```python
from build123d import *

# Parameters (mm, degrees)
F0_R      = 10
F1_DEPTH  = 2.5
F2_R      = 7.5
F3_DEPTH  = 10
F4_R      = 7.15
F5_DEPTH  = 1.5
F6_R      = 7.5
F7_DEPTH  = 16.5
F8_R      = 6
F9_DEPTH  = 20
F10_SIZE  = 1
F11_R     = 7.75
F12_DEPTH = 15
F13_R     = 2.75
F14_DEPTH = 42
F15_SIZE  = 1
F16_R     = 1.5
F17_DEPTH = 12.5
F19_DEPTH = 6
F20_DEPTH = 4.2


with BuildPart() as f1:
    # F0 (on Front) → F1 (new body, symmetric)
    with BuildSketch(Plane.XZ):
        Circle(F0_R)
    extrude(amount=F1_DEPTH, both=True)

    # F2 (on face) → F3 (join)
    with BuildSketch(Plane.XZ.offset(2.5)):
        Circle(F2_R)
    extrude(amount=F3_DEPTH)

    # F4 (on face) → F5 (join)
    with BuildSketch(Plane.XZ.offset(12.5)):
        Circle(F4_R)
    extrude(amount=F5_DEPTH)

    # F6 (on face) → F7 (join)
    with BuildSketch(Plane.XZ.offset(14)):
        Circle(F6_R)
    extrude(amount=F7_DEPTH)

    # F8 (on face) → F9 (join)
    with BuildSketch(Plane.XZ.offset(30.5)):
        Circle(F8_R)
    extrude(amount=F9_DEPTH)

    # F10
    f10_edges = [f1.edges().sort_by_distance(p)[0] for p in [
        (-6, -50.5, 0),
    ]]
    chamfer(f10_edges, length=F10_SIZE)

    # F11 (on face) → F12 (join)
    with BuildSketch(Plane(origin=(0, 2.5, 0), x_dir=(-1, 0, 0), z_dir=(0, 1, 0))):
        Circle(F11_R)
    extrude(amount=F12_DEPTH)

    # F13 (on face) → F14 (join)
    with BuildSketch(Plane(origin=(0, 17.5, 0), x_dir=(-1, 0, 0), z_dir=(0, 1, 0))):
        Circle(F13_R)
    extrude(amount=F14_DEPTH)

    # F15
    f15_edges = [f1.edges().sort_by_distance(p)[0] for p in [
        (2.75, 59.5, 0),
    ]]
    chamfer(f15_edges, length=F15_SIZE)

    # F16 (on Top) → F17 (cut, symmetric)
    with BuildSketch(Plane.XY):
        with Locations((0, 14.5)):
            Circle(F16_R)
    extrude(amount=F17_DEPTH, both=True, mode=Mode.SUBTRACT)

    # F18 (on Top) → F19 (cut)
    with BuildSketch(Plane.XY):
        with BuildLine():
            Line((-1.5, -34), (-1.5, -50.5))
            Line((-1.5, -50.5), (1.5, -50.5))
            Line((1.5, -50.5), (1.5, -34))
            ThreePointArc((1.5, -34), (1.06066, -32.93934), (0, -32.5))
            ThreePointArc((0, -32.5), (-1.06066, -32.93934), (-1.5, -34))
        make_face()
    extrude(amount=F19_DEPTH, mode=Mode.SUBTRACT)

    # F18 (on Top) → F20 (join)
    with BuildSketch(Plane.XY):
        with BuildLine():
            Line((-1.5, -34), (-1.5, -50.5))
            Line((-1.5, -50.5), (1.5, -50.5))
            Line((1.5, -50.5), (1.5, -34))
            ThreePointArc((1.5, -34), (1.06066, -32.93934), (0, -32.5))
            ThreePointArc((0, -32.5), (-1.06066, -32.93934), (-1.5, -34))
        make_face()
    extrude(amount=F20_DEPTH)


solid = f1.part
```
CAD build for the part. Positions are in the model's coordinates, mm. A direction names the side the tool comes from. Round coordinates to 2 decimals unless told otherwise and drop trailing zeros. Loops run counter-clockwise (first coordinate to the right, second up) from the corner with the lowest first, then second, coordinate; pieces in that order, holes last. Notation, with made-up numbers: M 34.5,22.5 L 71.5,22.5 A27 cw 71.5,46.5 Z; hole C 81.5,15 d4. An arc over 180 degrees is marked long. Return JSON: item names as keys, results as strings. Group by question number.
(1) Drop flat-ended pins along their axis: P1, Ø0.8, axis at y = -39, z = 5, coming from the +X side; P2, Ø12, axis at x = -6.5, y = 18, coming from the -Z side; P3, Ø2.5, axis at x = 0.5, y = -44, coming from the +Z side; P4, Ø1, axis at x = 4, y = 28.5, coming from the -Z side. Give the stop position or say it passes through.
(2) Wall check: probe 1 along X at (y, z) = (14.5, -2); probe 2 along Y at (x, z) = (0, -3); probe 3 along Y at (x, z) = (0, -1). Give the ranges that are in metal, low to high. Write a range as [from, to].
(3) Mould opens along Y. For faces 5 (the flat face through (2, -30.5, 6)), 6 (the cylindrical face through (-0.93, -13.24, 7.09)), 7 (the cylindrical face through (-2.17, -0.04, -9.76)) say: +Y half, -Y half, draft (parallel to the pull), parting line (faces both ways), or undercut.
(4) Tool access for faces 1 (the flat face through (0, -41, 4.2)), 2 (the cylindrical face through (1.68, 9.895, -7.566)), 3 (the flat face through (0, 59.5, 0)), 4 (the flat face through (4, -2.5, 7)): list every direction of +Z, -Z, +X, -X, +Y, -Y with a clear straight run to the whole face (end or side of a thin tool).
(5) Saw through at A-A, the plane y = 14.5. List the corners of the cut face in (x, z), and give its area (3 significant figures).
(6) Saw through at B-B, the plane y = -7. List the corners of the cut face in (x, z).
Answer list:
{
 "1": {"P1": "x = 3.85", "P2": "z = -7.73", "P3": "z = 5.81", "P4": "through"},
 "2": {"probe 1": "[-7.49, -1.5], [1.5, 7.49]", "probe 2": "[-50.5, 13], [16, 17.5]", "probe 3": "[-50.5, 13], [16, 59.5]"},
 "3": {"face 5": "-Y half", "face 6": "undercut", "face 7": "draft"},
 "4": {"face 1": "+Z, -Y", "face 2": "+Y", "face 3": "+Z, -Z, +X, -X, +Y", "face 4": "-Y"},
 "5": {"outline": "M -1.5,-7.6 L -1.5,7.6 A7.75 ccw Z; M 1.5,-7.6 A7.75 ccw 1.5,7.6 Z", "area": "142 mm2"},
 "6": {"outline": "C 0,0 d15"}
}
